Design review of the part shown in the three views and the two pictorial views. Dimensions are in mm from the part's minimum x, y and z. A direction names the side the tool comes from. Coordinates: 2 decimals unless noted, no trailing zeros. Loops run counter-clockwise (first coordinate to the right, second up) from the corner with the lowest first, then second, coordinate; pieces in that order, holes last. Notation, with made-up numbers: M 64.5,59.5 L 91.5,59.5 A6 ccw 91.5,65.5 Z; hole C 63.5,44 d5. An arc over 180 degrees is marked long. Answer as a JSON object with one key per item and string values. Group by question number.
Item 1: Insertion check: pin 1 (22.5 mm diameter, centred on x = 20, y = 20, fed in from -Z); pin 2 (4.5 mm diameter, centred on x = 36.5, y = 20, fed in from -Z); pin 3 (2 mm diameter, centred on x = 19.5, y = 21, fed in from +Z). Each pin has a flat end and moves straight along its axis. Give the tip position at first contact, or say it passes through.
Item 2: Add section C-C (y = 5). State the section outline as (x, z) points.
Item 3: Add section A-A (y = 20). State the section outline as (x, z) points, then the cut area to 3 significant figures.
Item 4: Wall thickness on L1, parallel to Y at x = 3.5, z = 13; L2, parallel to Y at x = 36.5, z = 6.65; L3, parallel to Z at x = 25, y = 11: over which ranges is each line inside the solid? List them lowest first. Write a range as from..to.
Item 5: Mouldability with a two-part tool opening along X and no side actions: class the marked faces 3, 4 and 5 as +X half, -X half, draft (parallel to the pull), parting line (faces both ways), or undercut.
Item 6: Tool access review of the marked faces 1 and 2: name each direction out of +Z, -Z, +X, -X, +Y, -Y from which nothing blocks a thin tool from reaching the whole face with its end or side.
Item 7: Add section B-B (z = 7.75). State the section outline as (x, y) points, then the cut area to 3 significant figures.
Item 8: Add section D-D (x = 29). State the section outline as (y, z) points, then the cut area to 3 significant figures.
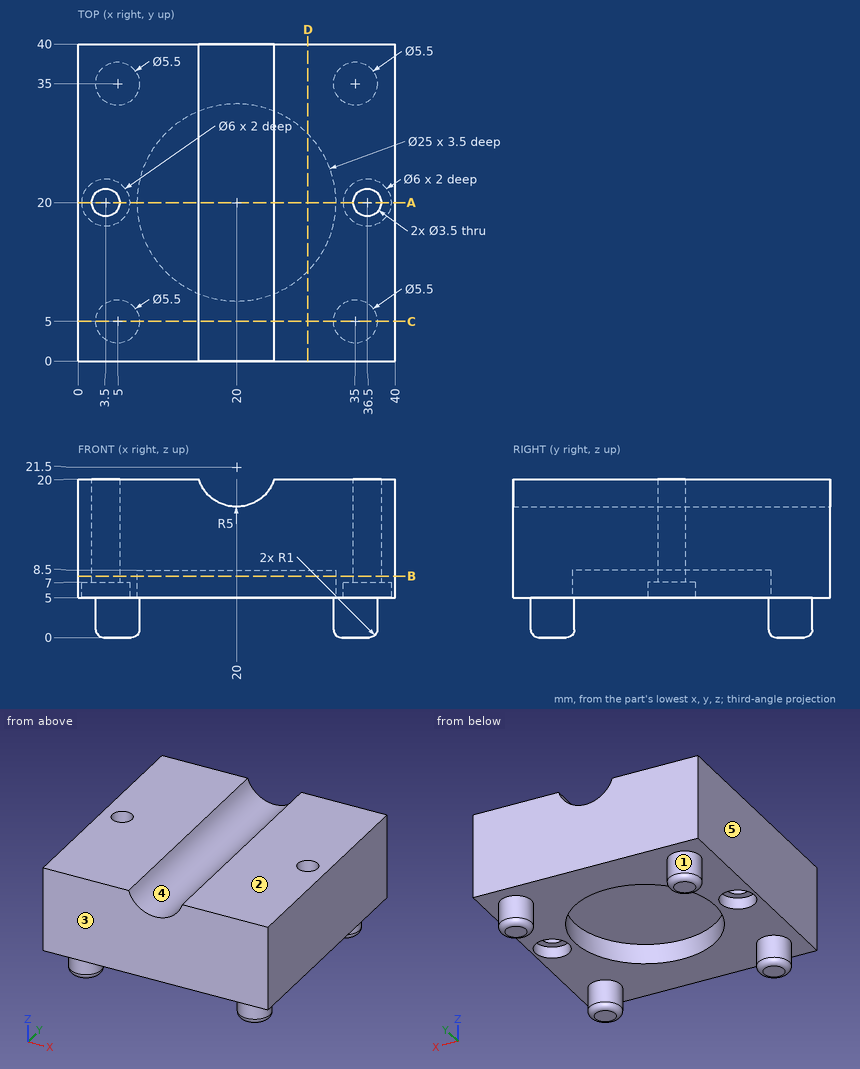
From the geometry:
{
 "1": {"pin 1": "stops at z = 8.5", "pin 2": "stops at z = 7", "pin 3": "stops at z = 16.73"},
 "2": {"outline": "M 0,5 L 2.25,5 L 2.25,1 A1 ccw 3.25,0 L 6.75,0 A1 ccw 7.75,1 L 7.75,5 L 32.25,5 L 32.25,1 A1 ccw 33.25,0 L 36.75,0 A1 ccw 37.75,1 L 37.75,5 L 40,5 L 40,20 L 24.77,20 A5 cw 15.23,20 L 0,20 Z"},
 "3": {"outline": "M 0,5 L 0.5,5 L 0.5,7 L 1.75,7 L 1.75,20 L 0,20 Z; M 5.25,7 L 6.5,7 L 6.5,5 L 7.5,5 L 7.5,8.5 L 32.5,8.5 L 32.5,5 L 33.5,5 L 33.5,7 L 34.75,7 L 34.75,20 L 24.77,20 A5 cw 15.23,20 L 5.25,20 Z; M 38.25,7 L 39.5,7 L 39.5,5 L 40,5 L 40,20 L 38.25,20 Z", "area": "373 mm²"},
 "4": {"L1": "y = 0..18.25, 21.75..40", "L2": "y = 0..17, 23..40", "L3": "z = 8.5..20"},
 "5": {"face 3": "draft", "face 4": "undercut", "face 5": "-X half"},
 "6": {"face 1": "-Z", "face 2": "+Z, +X, -X, +Y, -Y"},
 "7": {"outline": "M 0,0 L 40,0 L 40,40 L 0,40 Z; hole C 3.5,20 d3.5; hole C 20,20 d25; hole C 36.5,20 d3.5", "area": "1,090 mm²"},
 "8": {"outline": "M 0,5 L 11.33,5 L 11.33,8.5 L 28.67,8.5 L 28.67,5 L 40,5 L 40,20 L 0,20 Z", "area": "539 mm²"}
}
